Input: part model. Units: mm. Frame: model coordinates. A direction names the side the tool comes from. Coordinates: 2 decimals unless noted, no trailing zeros. Loops run counter-clockwise (first coordinate to the right, second up) from the corner with the lowest first, then second, coordinate; pieces in that order, holes last.
Item 1: Section C-C on y = 20. Return loops of the section in (x, z).
Item 2: Ray query, line 1 along X through (y, z) = (17.5, 2.5); line 2 along X through (y, z) = (-2, 6.5); line 3 along X through (y, z) = (1, 1). Return the intervals inside material, ascending.
Item 3: Section B-B on z = 17. Return loops of the section in (x, y).
Item 4: Section A-A on x = 8. Return loops of the section in (y, z), and give its area (4 significant figures).
Item 5: Reachability of faces 1 (the flat face through (12.5, 8, 11)), 2 (the flat face through (26, -17.9, 2)), 3 (the flat face through (-28, -8, 21)), 4 (the cylindrical face through (-0.04, 27.25, 2.46)), 5 (the flat face through (-26, -23.1, 2)) from +Z, -Z, +X, -X, +Y, -Y: full face, straight path, thin tool, end or side. Return the list, or none.
Item 6: Contact query for flat-ended pins moving along their axis: P1, Ø2, axis at y = 16.5, z = 2.5, coming from the +X side; P2, Ø2, axis at x = 4.5, y = -14.5, coming from the +Z side; P3, Ø2, axis at y = -1.5, z = 4.5, coming from the -X side; P4, Ø8, axis at x = -3, y = 12.5, coming from the -Z side. Output: stop coordinate, or through.
Item 7: Section D-D on x = 14.5. Return loops of the section in (y, z), and give its area (3 significant figures).
Item 8: Pull-direction query (X, two-part tool) for faces 6 (the flat face through (29.5, -8, 6)), 7 (the cylindrical face through (8.04, 13.75, 2.46)), 8 (the flat face through (0, 30.5, 2)); classes: released by +X, released by -X, zero draft, split by the parting line, or undercut.
```python
from build123d import *

# Parameters (mm, degrees)
BOSS_EXTRUDE1_DEPTH = 5
BOSS_EXTRUDE2_DEPTH = 16
CUT_EXTRUDE1_DEPTH  = 60.835190315
CUT_EXTRUDE2_DEPTH  = 16
FILLET1_R           = 1
FILLET2_R           = 1


with BuildPart() as part:
    # Sketch1 → Boss-Extrude1 (new body)
    with BuildSketch(Plane.XY):
        with BuildLine():
            Line((-29.5, -23.1), (-29.5, -30.5))
            Line((-29.5, -30.5), (29.5, -30.5))
            Line((29.5, -30.5), (29.5, -23.1))
            Line((29.5, -23.1), (22, -23.1))
            ThreePointArc((22, -23.1), (19.4, -20.5), (22, -17.9))
            Line((22, -17.9), (29.5, -17.9))
            Line((29.5, -17.9), (29.5, -5.5))
            Line((29.5, -5.5), (17.5, -5.5))
            Line((17.5, -5.5), (17.5, 30.5))
            Line((17.5, 30.5), (-17.5, 30.5))
            Line((-17.5, 30.5), (-17.5, -5.5))
            Line((-17.5, -5.5), (-29.5, -5.5))
            Line((-29.5, -5.5), (-29.5, -17.9))
            Line((-29.5, -17.9), (-22, -17.9))
            ThreePointArc((-22, -17.9), (-19.4, -20.5), (-22, -23.1))
            Line((-22, -23.1), (-29.5, -23.1))
        make_face()
        with BuildLine():
            ThreePointArc((-9.75, 17.5), (-8, 19.25), (-6.25, 17.5))
            Line((-6.25, 17.5), (-6.25, 15.5))
            ThreePointArc((-6.25, 15.5), (-8, 13.75), (-9.75, 15.5))
            Line((-9.75, 15.5), (-9.75, 17.5))
        make_face(mode=Mode.SUBTRACT)
        with BuildLine():
            ThreePointArc((-1.75, 25.5), (0, 27.25), (1.75, 25.5))
            Line((1.75, 25.5), (1.75, 22.714163404))
            ThreePointArc((1.75, 22.714163404), (4.465142775, 20.711308145), (5.5, 17.5))
            Line((5.5, 17.5), (5.5, 15.5))
            ThreePointArc((5.5, 15.5), (4.465142775, 12.288691855), (1.75, 10.285836596))
            Line((1.75, 10.285836596), (1.75, 7.5))
            ThreePointArc((1.75, 7.5), (0, 5.75), (-1.75, 7.5))
            Line((-1.75, 7.5), (-1.75, 10.285836596))
            ThreePointArc((-1.75, 10.285836596), (-4.465142775, 12.288691855), (-5.5, 15.5))
            Line((-5.5, 15.5), (-5.5, 17.5))
            ThreePointArc((-5.5, 17.5), (-4.465142775, 20.711308145), (-1.75, 22.714163404))
            Line((-1.75, 22.714163404), (-1.75, 25.5))
        make_face(mode=Mode.SUBTRACT)
        with BuildLine():
            Line((6.25, 15.5), (6.25, 17.5))
            ThreePointArc((6.25, 17.5), (8, 19.25), (9.75, 17.5))
            Line((9.75, 17.5), (9.75, 15.5))
            ThreePointArc((9.75, 15.5), (8, 13.75), (6.25, 15.5))
        make_face(mode=Mode.SUBTRACT)
    extrude(amount=BOSS_EXTRUDE1_DEPTH)

    # Sketch2 → Boss-Extrude2 (add)
    with BuildSketch(Plane.XY.offset(5)):
        Polygon((-17.5, 30.5), (-12.5, 30.5), (-12.5, -5.5), (12.5, -5.5), (12.5, 30.5), (17.5, 30.5), (17.5, -5.5), (29.5, -5.5), (29.5, -10.5), (-29.5, -10.5), (-29.5, -5.5), (-17.5, -5.5), align=None)
    extrude(amount=BOSS_EXTRUDE2_DEPTH)

    # Sketch3 → Cut-Extrude1 (cut, through all)
    with BuildSketch(Plane(origin=(17.5, 0, 0), x_dir=(0, 0, -1), z_dir=(1, 0, 0))):
        Polygon((-21, -5.5), (-21, 30.5), (-5, 30.5), align=None)
    extrude(amount=-CUT_EXTRUDE1_DEPTH, mode=Mode.SUBTRACT)

    # Sketch4 → Cut-Extrude2 (cut)
    with BuildSketch(Plane.XZ.offset(10.5)):
        with BuildLine():
            Line((-26.1, 15), (-26.1, 21))
            Line((-26.1, 21), (-20.9, 21))
            Line((-20.9, 21), (-20.9, 15))
            ThreePointArc((-20.9, 15), (-23.5, 12.4), (-26.1, 15))
        make_face()
        with BuildLine():
            Line((20.9, 21), (20.9, 15))
            ThreePointArc((20.9, 15), (23.5, 12.4), (26.1, 15))
            Line((26.1, 15), (26.1, 21))
            Line((26.1, 21), (20.9, 21))
        make_face()
    extrude(amount=-CUT_EXTRUDE2_DEPTH, mode=Mode.SUBTRACT)

    # Fillet1
    fillet1_edges = [part.edges().sort_by_distance(p)[0] for p in [
        (-29.5, -10.5, 13),
        (29.5, -10.5, 13),
        (-17.5, 30.5, 2.5),
        (17.5, 30.5, 2.5),
        (29.5, -30.5, 2.5),
        (-29.5, -30.5, 2.5),
        (-29.5, -5.5, 10.5),
        (29.5, -5.5, 10.5),
    ]]
    fillet(fillet1_edges, radius=FILLET1_R)

    # Fillet2
    fillet2_edges = [part.edges().sort_by_distance(p)[0] for p in [
        (-1.75, 10.285836596, 2.5),
        (1.75, 10.285836596, 2.5),
        (1.75, 22.714163404, 2.5),
        (-1.75, 22.714163404, 2.5),
    ]]
    fillet(fillet2_edges, radius=FILLET2_R)


solid = part.part
```
Results found:
1. outline: (-17.5, 0) - (-4.9, 0) - (-4.9, 5) - (-12.5, 5) - (-12.5, 9.67) - (-17.5, 9.67) - close; (4.9, 0) - (17.5, 0) - (17.5, 9.67) - (12.5, 9.67) - (12.5, 5) - (4.9, 5) - close
2. line 1: x = -17.5 to -9.75, -6.25 to -5.5, 5.5 to 6.25, 9.75 to 17.5
2. line 2: x = -17.5 to -12.5, 12.5 to 17.5
2. line 3: x = -17.5 to 17.5
3. outline: (-29.5, -9.5) arc R1 ccw to (-28.5, -10.5) - (-26.1, -10.5) - (-26.1, -5.5) - (-28.5, -5.5) arc R1 ccw to (-29.5, -6.5) - close; (-20.9, -10.5) - (20.9, -10.5) - (20.9, -5.5) - (17.5, -5.5) - (17.5, 3.5) - (12.5, 3.5) - (12.5, -5.5) - (-12.5, -5.5) - (-12.5, 3.5) - (-17.5, 3.5) - (-17.5, -5.5) - (-20.9, -5.5) - close; (26.1, -10.5) - (28.5, -10.5) arc R1 ccw to (29.5, -9.5) - (29.5, -6.5) arc R1 ccw to (28.5, -5.5) - (26.1, -5.5) - close
4. outline: (-30.5, 0) - (13.75, 0) - (13.75, 5) - (-5.5, 5) - (-5.5, 21) - (-10.5, 21) - (-10.5, 5) - (-30.5, 5) - close; (19.25, 0) - (30.5, 0) - (30.5, 5) - (19.25, 5) - close
4. area: 357.5 mm2
5. face 1: +Z, +Y
5. face 2: +Z, -Z, +X
5. face 3: +Z, +X, -X, +Y, -Y
5. face 4: +Z, -Z
5. face 5: +Z, -Z, -X
6. P1: stops at x = 17.5
6. P2: stops at z = 5
6. P3: stops at x = -17.5
6. P4: stops at z = 0
7. outline: (-30.5, 0) - (30.5, 0) - (30.5, 5) - (-5.5, 21) - (-10.5, 21) - (-10.5, 5) - (-30.5, 5) - close
7. area: 673 mm2
8. face 6: released by +X
8. face 7: undercut
8. face 8: zero draft
